Can you work these out from the drawing? Everything is in mm from the part's minimum corner. A direction names the side the tool comes from. Round coordinates to 2 decimals unless told otherwise and drop trailing zeros. Loops run counter-clockwise (first coordinate to the right, second up) from the corner with the lowest first, then second, coordinate; pieces in that order, holes last. Notation, with made-up numbers: M 56.25,76 L 77.25,76 A21 cw 77.25,105 Z; hole C 33,86 d2. An arc over 180 degrees is marked long. Use a Markdown table: item, result.
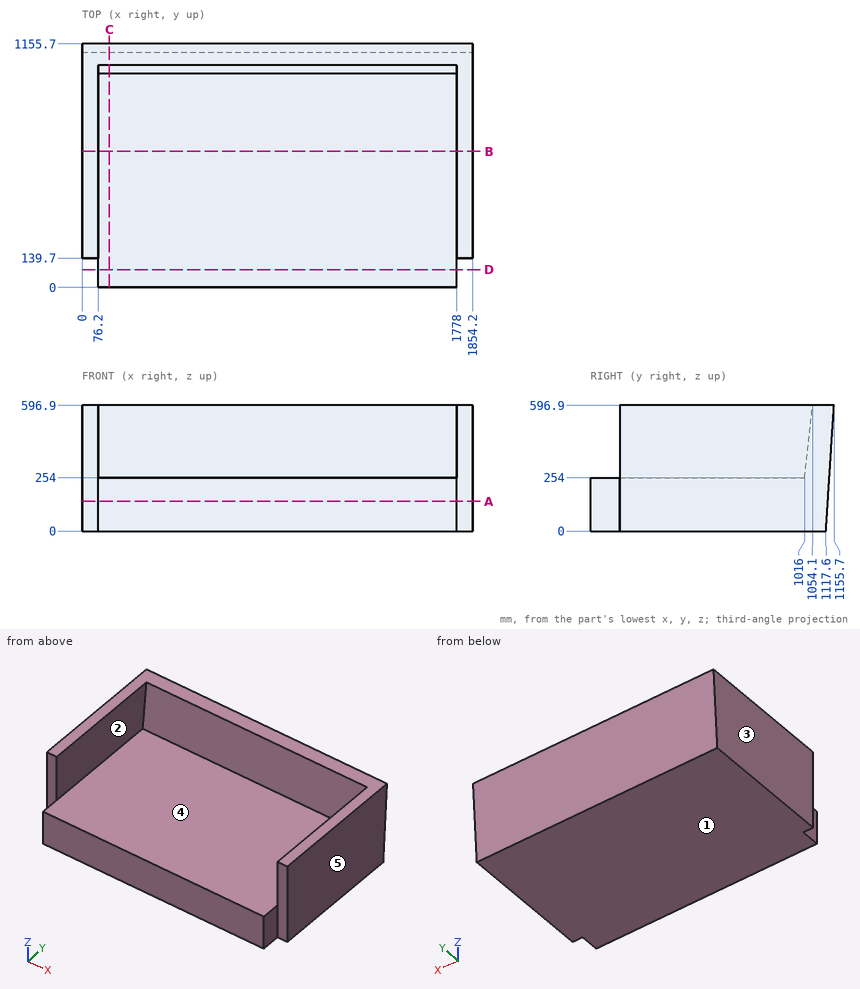
Q1. We'd pull the mould along X, two halves only. Please class the marked faces 1, 2 and 3: pulls with the +X half, pulls with the -X half, needs draft (parallel to the pull), parting line crosses it, or undercut.
Return value:
| item | result |
|---|---|
| face 1 | needs draft |
| face 2 | undercut |
| face 3 | pulls with the -X half |
Q2. Imagine slicing it at D-D, the plane y = 85. Please give me the cut outline in (x, z).
Return value:
| item | result |
|---|---|
| outline | M 76.2,0 L 1778,0 L 1778,254 L 76.2,254 Z |
Q3. For the marked faces 4 and 5, which set-ups out of +Z, -Z, +X, -X, +Y, -Y let a thin tool reach every point of the face, with its end or its side?
Return value:
| item | result |
|---|---|
| face 4 | +Z, -Y |
| face 5 | +Z, -Z, +X, +Y, -Y |
Q4. Will these pins go through, and if not, where does the flat tip stop? P1, Ø5, axis at x = 1147.5, y = 667, coming from the -Z side; P2, Ø10, axis at x = 993.5, y = 510.5, coming from the +Z side; P3, Ø4, axis at x = 1500.5, z = 519, coming from the -Y side.
Return value:
| item | result |
|---|---|
| P1 | stops at z = 0 |
| P2 | stops at z = 254 |
| P3 | stops at y = 1045.22 |
Q5. Imagine slicing it at C-C, the plane x = 130. Please give me the cut outline in (y, z).
Return value:
| item | result |
|---|---|
| outline | M 0,0 L 1117.6,0 L 1155.7,596.9 L 1054.1,596.9 L 1016,254 L 0,254 Z |
Q6. Imagine slicing it at A-A, the plane z = 141. Please give me the cut outline in (x, y).
Return value:
| item | result |
|---|---|
| outline | M 0,139.7 L 76.2,139.7 L 76.2,0 L 1778,0 L 1778,139.7 L 1854.2,139.7 L 1854.2,1126.6 L 0,1126.6 Z |
Q7. I need wall thicknesses on line 1 (X direction, y = 324, z = 314); line 2 (Z direction, x = 1166, y = 112); line 3 (X direction, y = 96, z = 193.5). Which ranges of each line are inside material? Lowest first, please. Write a range as from..to.
Return value:
| item | result |
|---|---|
| line 1 | x = 0..76.2, 1778..1854.2 |
| line 2 | z = 0..254 |
| line 3 | x = 76.2..1778 |
Q8. Imagine slicing it at B-B, the plane y = 646.5. Please give me the cut outline in (x, z), then the cut area to 3 significant figures.
Return value:
| item | result |
|---|---|
| outline | M 0,0 L 1854.2,0 L 1854.2,596.9 L 1778,596.9 L 1778,254 L 76.2,254 L 76.2,596.9 L 0,596.9 Z |
| area | 523,000 mm^2 |
